```python
from build123d import *

# Parameters (mm, degrees)
SKETCH_1_R      = 1.5
EXTRUDE_1_DEPTH = 1.4
SKETCH_4_W      = 4
SKETCH_4_H      = 1.4
EXTRUDE_2_DEPTH = 4.5
SKETCH_5_R      = 3.25
SKETCH_5_R_2    = 1.85
EXTRUDE_3_DEPTH = 4.5
FILLET_1_R      = 1


with BuildPart() as part:
    # 草图1 → 凸台-拉伸1 (new body)
    with BuildSketch(Plane.XY):
        with BuildLine():
            Line((-2, -10), (2, -10))
            ThreePointArc((2, -10), (2.707106781, -9.707106781), (3, -9))
            Line((3, -9), (3, 9))
            ThreePointArc((3, 9), (2.707106781, 9.707106781), (2, 10))
            Line((2, 10), (-2, 10))
            ThreePointArc((-2, 10), (-2.707106781, 9.707106781), (-3, 9))
            Line((-3, 9), (-3, -9))
            ThreePointArc((-3, -9), (-2.707106781, -9.707106781), (-2, -10))
        make_face()
        with Locations((0, 6)):
            Circle(SKETCH_1_R, mode=Mode.SUBTRACT)
        with Locations(Location((0, -6, 0), (0, 0, 180))):
            Circle(SKETCH_1_R, mode=Mode.SUBTRACT)
    extrude(amount=EXTRUDE_1_DEPTH)

    # 草图4 → 凸台-拉伸2 (add)
    with BuildSketch(Plane(origin=(0, -9, 0), x_dir=(-1, 0, 0), z_dir=(0, -1, 0))):
        with Locations((-5, -0.7)):
            Rectangle(SKETCH_4_W, SKETCH_4_H)
    extrude_2 = extrude(amount=-EXTRUDE_2_DEPTH)

    # 草图5 → 凸台-拉伸3 (add)
    with BuildSketch(Plane.XZ.offset(9)):
        with Locations((7, -1.85)):
            Circle(SKETCH_5_R)
        with Locations(Location((7, -1.85, 0), (0, 0, 270))):
            Circle(SKETCH_5_R_2, mode=Mode.SUBTRACT)
    extrude_3 = extrude(amount=-EXTRUDE_3_DEPTH)

    # 镜向1: 凸台-拉伸2, 凸台-拉伸3 across plane
    add(extrude_2.mirror(Plane.ZX.offset(-2.25)))
    add(extrude_3.mirror(Plane.ZX.offset(-2.25)))

    # 圆角1
    fillet_1_edges = [part.edges().sort_by_distance(p)[0] for p in [
        (3, -9, 0.7),
        (3, -4.5, 0.7),
        (3, 4.5, 0.7),
        (3, 0, 0.7),
    ]]
    fillet(fillet_1_edges, radius=FILLET_1_R)


solid = part.part
```
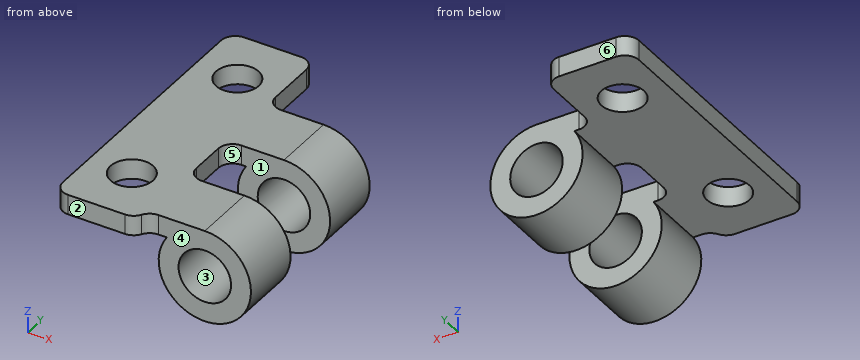
For this review, take the finished solid that the model builds, in its own axes (mm). Face numbers are marked on the shaded views. A direction names the side the tool comes from. Round coordinates to 2 decimals unless told otherwise and drop trailing zeros. Loops run counter-clockwise (first coordinate to the right, second up) from the corner with the lowest first, then second, coordinate; pieces in that order, holes last.
Q1. To check wall thickness, follow line 1 along Y through (x, z) = (0, 1); line 2 along Y through (x, z) = (4, -1.5); line 3 along X through (y, z) = (2.25, -1.85). State the ranges of each line that lie inside material, in increasing order.
Result sheet:
line 1: y = -10 to -7.5, -4.5 to 4.5, 7.5 to 10
line 2: y = -9 to -4.5, 0 to 4.5
line 3: x = 3.75 to 5.15, 8.85 to 10.25
Q2. Add section A-A on y = -6. Write out the cut boundary in (x, z), plus the area to 3 significant figures.
Result sheet:
outline: (-3, 0) - (-1.5, 0) - (-1.5, 1.4) - (-3, 1.4) - close; (1.5, 0) - (4.33, 0) arc R3.25 ccw (long way) to (7, 1.4) - (1.5, 1.4) - close; hole circle Ø3.7 at (7, -1.85)
area: 29.6 mm2
Q3. Add section C-C on x = 0. Write out the cut boundary in (y, z), plus the area to 3 significant figures.
Result sheet:
outline: (-10, 0) - (-7.5, 0) - (-7.5, 1.4) - (-10, 1.4) - close; (-4.5, 0) - (4.5, 0) - (4.5, 1.4) - (-4.5, 1.4) - close; (7.5, 0) - (10, 0) - (10, 1.4) - (7.5, 1.4) - close
area: 19.6 mm2
Q4. Add section D-D on z = -1.85. Write out the cut boundary in (x, y), plus the area to 3 significant figures.
Result sheet:
outline: (3.75, -9) - (5.15, -9) - (5.15, -4.5) - (3.75, -4.5) - close; (3.75, 0) - (5.15, 0) - (5.15, 4.5) - (3.75, 4.5) - close; (8.85, -9) - (10.25, -9) - (10.25, -4.5) - (8.85, -4.5) - close; (8.85, 0) - (10.25, 0) - (10.25, 4.5) - (8.85, 4.5) - close
area: 25.2 mm2
Q5. Insertion check: pin 1 Ø5 at (x, y) = (0, 6) entering from -Z; pin 2 Ø1.5 at (y, z) = (-3.5, 0) entering from +X; pin 3 Ø3 at (x, z) = (8, -1.5) entering from +Y. Each pin has a flat end and moves straight along its axis. Give the tip position at first contact, or say it passes through.
Result sheet:
pin 1: stops at z = 0
pin 2: stops at x = 3.34
pin 3: stops at y = 4.5
Q6. Machinability: for the marked faces 4, 5 and 6, which of the approach directions +Z, -Z, +X, -X, +Y, -Y give a long, thin tool a straight path to every point of the face, cutting with its end or side? Answer none if there is none.
Result sheet:
face 4: +Z, -Z, +X, -Y
face 5: +Z, -Z, +X
face 6: +Z, -Z, +X, -X, +Y
Q7. Mouldability with a two-part tool opening along Y and no side actions: class the marked faces 1, 2 and 3 as +Y half, -Y half, draft (parallel to the pull), parting line (faces both ways), or undercut.
Result sheet:
face 1: undercut
face 2: -Y half
face 3: draft
Q8. Add section B-B on y = 6. Write out the cut boundary in (x, z).
Result sheet:
outline: (-3, 0) - (-1.5, 0) - (-1.5, 1.4) - (-3, 1.4) - close; (1.5, 0) - (3, 0) - (3, 1.4) - (1.5, 1.4) - close
